Autodesk Inventor part; units mm, degrees
ref_plane "YZ Plane" through (0, 0, 0) normal (1, 0, 0) x (0, 1, 0)
ref_plane "XZ Plane" through (0, 0, 0) normal (0, 1, 0) x (-1, 0, 0)
ref_plane "XY Plane" through (0, 0, 0) normal (0, 0, 1) x (1, 0, 0)
sketch "Sketch1" plane through (0, 0, 0) normal (0, 1, 0) x (-1, 0, 0)
  line L0 (5.3848, 9.7652) -> (-6.6152, 9.7652)
  line L1 (-6.6152, 9.7652) -> (-6.6152, 5.2652)
  line L2 (-6.6152, 5.2652) -> (5.3848, 5.2652)
  line L3 (5.3848, 5.2652) -> (5.3848, 9.7652)
  point P0 (0, 0)
  dimension "d0" = 12
  dimension "d1" = 4.5
extrude "Extrusion1" add sketch "Sketch1" along normal blind 27
shell "Shell1" thickness 0.2 removed faces 2 at (2.6152, 27, 8.2652) at (2.6152, 0, 8.2652)
sketch "Sketch2" plane through (6.6152, 0, 9.7652) normal (1, 0, 0) x (0, 0, -1)
  line L0 (0, 0) -> (0, 27)
  line L1 (0, 27) -> (0, 15)
  line L2 (0, 15) -> (0.2, 15)
  line L3 (0.2, 15) -> (0.2, 16)
  line L4 (0, 27) -> (0.2, 27)
  line L5 (0.2, 27) -> (0.2, 26)
  line L6 (0.2, 27) -> (4.3, 27)
  line L7 (0.2, 26) -> (2.25, 23.95)
  line L8 (0.2, 16) -> (2.25, 18.05)
  line L9 (2.25, 18.05) -> (2.25, 23.95)
  line L10 (0, 0) -> (0, 27)
  point P0 (9.7652, 0)
  dimension "d5" = 12
  dimension "d6" = 0.2
  dimension "d7" = 1
  dimension "d9" = 1
  dimension "d12" = 2.05
  dimension "d15" = 2.05
  dimension "d16" = 5.9
  dimension "d17" = 2.05
extrude "Extrusion2" cut sketch "Sketch2" against normal up to next
sketch "Sketch3" plane through (-5.1848, 0, 5.4652) normal (0, 0, 1) x (1, 0, 0)
  circle A0 centre (2.8, 23.3) radius 1.5
  circle A1 centre (8.8, 23.3) radius 1.5
  line L0 (0, 27) -> (11.6, 27)
  line L1 (-0.2, 23.95) -> (-0.2, 26)
  line L2 (11.8, 26) -> (11.8, 23.95)
  point P0 (5.1848, 0)
  dimension "d20" = 3
  dimension "d21" = 3.7
  dimension "d22" = 3
  dimension "d23" = 3
extrude "Extrusion3" cut sketch "Sketch3" against normal up to next
sketch "Sketch4" plane through (0, 0, 0) normal (0, -1, 0) x (1, 0, 0)
  line L0 (-5.1848, 9.5652) -> (-5.3848, 9.5652)
  line L1 (-5.1848, 9.5652) -> (6.4152, 9.5652)
  line L2 (6.4152, 9.5652) -> (6.4152, 8.0652)
  line L3 (6.4152, 8.0652) -> (-5.1848, 8.0652)
  line L4 (-5.1848, 8.0652) -> (-5.1848, 9.5652)
  point P0 (0, 0)
  dimension "d26" = 11.6
  dimension "d27" = 1.5
extrude "Extrusion4" add sketch "Sketch4" along normal blind 1 and the other way blind 14.5
move faces "Move1" translate (0, 1.5, 0) faces at (-1.3181, -1, 9.0652)
properties part number "USB_Contact"
Part model, mm, in its own coordinate system. A direction names the side the tool comes from. Round coordinates to 2 decimals unless told otherwise and drop trailing zeros. Write each loop counter-clockwise with the first axis right and the second up, starting at its lowest first coordinate (ties: lowest second). Pieces come first, ordered by that corner, then holes.
Item 1: Probe L1, parallel to Z at x = -4.25, y = 10; L2, parallel to X at y = 7.5, z = 7.75; L3, parallel to Y at x = -1.5, z = 9.45. List the from-to ranges inside material, lowest first.
Results:
L1: z = 5.27 to 5.47, 8.07 to 9.77
L2: x = -5.38 to -5.18, 6.42 to 6.62
L3: y = 0.5 to 14.5
Item 2: Drop flat-ended pins along their axis: pin 1 Ø1.5 at (x, z) = (-0.5, 7.5) entering from -Y; pin 2 Ø2 at (x, z) = (3, 6.5) entering from -Y. Give the stop position or say it passes through.
Results:
pin 1: stops at y = 0.5
pin 2: passes through
Item 3: Cut at D-D, the plane y = 9. Give the cut face in (x, z), plus the area to 3 significant figures.
Results:
outline: (-5.38, 5.27) - (6.62, 5.27) - (6.62, 9.77) - (-5.38, 9.77) - close; hole (-5.18, 5.47) - (6.42, 5.47) - (6.42, 8.07) - (-5.18, 8.07) - close
area: 23.8 mm2
Item 4: Cut at B-B, the plane x = 0.5. Give the cut face in (y, z), plus the area to 3 significant figures.
Results:
outline: (0, 5.27) - (27, 5.27) - (27, 5.47) - (0, 5.47) - close; (0, 9.57) - (0.5, 9.57) - (0.5, 8.07) - (14.5, 8.07) - (14.5, 9.57) - (15, 9.57) - (15, 9.77) - (0, 9.77) - close
area: 29.4 mm2
Item 5: Which spindle directions (+Z, -Z, +X, -X, +Y, -Y) get a long thin tool onto all of the face, cutting with end or side? Do faces 1 (the flat face through (1, 13, 5.465)), 2 (the flat face through (1, 0.5, 9)), 3 (the flat face through (-5.385, 13, 7)). Say none if no direction does.
Results:
face 1: +Y, -Y
face 2: -Y
face 3: +Z, -Z, -X, +Y, -Y
Item 6: Cut at C-C, the plane z = 6.75. Give the cut face in (x, y).
Results:
outline: (-5.38, 0) - (-5.18, 0) - (-5.18, 27) - (-5.38, 27) - close; (6.42, 0) - (6.62, 0) - (6.62, 27) - (6.42, 27) - close
Item 7: Two-plate mould, pull along X, no slides. Class faces 4 (the flat face through (1, 7, 9.765)), 5 (the flat face through (6.615, 13, 8)), 6 (the flat face through (1, 14.5, 9)): +X half, -X half, draft (parallel to the pull), parting line (faces both ways), or undercut.
Results:
face 4: draft
face 5: +X half
face 6: undercut
Item 8: Cut at A-A, the plane y = 23.3. Give the cut face in (x, z).
Results:
outline: (-5.38, 5.27) - (-3.88, 5.27) - (-3.88, 5.47) - (-5.18, 5.47) - (-5.18, 7.52) - (-5.38, 7.52) - close; (-0.88, 5.27) - (2.12, 5.27) - (2.12, 5.47) - (-0.88, 5.47) - close; (5.12, 5.27) - (6.62, 5.27) - (6.62, 7.52) - (6.42, 7.52) - (6.42, 5.47) - (5.12, 5.47) - close
